Here's how the part is built. I have some questions about the finished solid (model axes, mm). A direction names the side the tool comes from. Round coordinates to 2 decimals unless told otherwise and drop trailing zeros. Order: outer loops, then holes, each group sorted by start corner. A loop starts at its lowest first (then second) coordinate and runs counter-clockwise, first axis right, second up. Notation, with made-up numbers: (17.5, 6.5) -> (46.5, 6.5) arc R13 cw to (46.5, 15.5) -> close; hole circle Ø7 at (70, 9). An arc over 180 degrees is marked (long way). Use a Markdown table: item, result. Add a question column.
(1) I want a section at D-D, the plane z = 25.5. Give the number of separate pieces and of enclosed holes in the cut face, then the cut area to 3 significant figures.
(2) On a 3-axis mill with a long thin cutter (end or side, diameter ignored), from which of +Z, -Z, +X, -X, +Y, -Y can I reach the whole of each face in a straight line? I mean faces 4 (the face through (7, 42, 28)), 5 (the face through (0, 32, 13)), 6 (the face through (2, 12, 28)), 7 (the face through (13, 36, 24)), 8 (the face through (5, 11, 14)). Say none if no direction works.
(3) I want a section at A-A, the plane z = 38. Please give me the cut outline in (x, y), then the cut area to 3 significant figures.
(4) Thinking about a two-plate mould opening in X: for faces 1 (the face through (2, 0, 14)), 2 (the face through (18.642, 25.535, 35.273)), 3 (the face through (15, 38, 26)), which applies, pulls with the +X half, pulls with the -X half, needs draft (parallel to the pull), parting line crosses it, or undercut?
(5) If I drill on probe 1 along Z at (x, y) = (3.95, 60); probe 2 along X at (y, z) = (26, 38); probe 3 along Z at (x, y) = (19, 25.45), over which ranges is the centre line in solid material (lowest first)?
(6) I want a section at B-B, the plane y = 60. Please give me the cut outline in (x, z).
(7) I want a section at C-C, the plane x = 20.5. Please give me the cut outline in (y, z), then the cut area to 3 significant figures.
(8) I'm going to push flat-ended pins straight in: P1, Ø11.5, axis at y = 14, z = 7, coming from the +X side; P2, Ø4, axis at x = 9, z = 24, coming from the -Y side; P3, Ø4, axis at x = 7.5, z = 19.5, coming from the +Y side. Where does each tip first touch, or does it pass through?
Autodesk Inventor part; units mm, degrees
ref_plane "YZ Plane" through (0, 0, 0) normal (1, 0, 0) x (0, 1, 0)
ref_plane "XZ Plane" through (0, 0, 0) normal (0, 1, 0) x (-1, 0, 0)
ref_plane "XY Plane" through (0, 0, 0) normal (0, 0, 1) x (1, 0, 0)
sketch "Sketch1" plane through (0, 0, 0) normal (1, 0, 0) x (0, 1, 0)
  line L0 (0, 0) -> (64, 0)
  line L1 (64, 0) -> (64, 28)
  line L2 (64, 28) -> (0, 28)
  line L3 (0, 28) -> (0, 0)
  line L4 (60, 24.5) -> (4, 24.5) construction
  line L5 (4, 24.5) -> (4, 3.5) construction
  line L6 (4, 3.5) -> (60, 3.5) construction
  line L7 (60, 3.5) -> (60, 24.5) construction
  line L8 (60, 24.5) -> (64, 24.5) construction
  line L9 (60, 24.5) -> (60, 28) construction
  line L10 (4, 3.5) -> (0, 3.5) construction
  line L11 (4, 3.5) -> (4, 0) construction
  circle A0 centre (60, 24.5) radius 2.6
  circle A1 centre (60, 3.5) radius 2.6
  circle A2 centre (4, 3.5) radius 2.6
  circle A3 centre (4, 24.5) radius 2.6
  dimension "d0" = 64
  dimension "d1" = 28
  dimension "d2" = 56
  dimension "d3" = 21
  dimension "d4" = 5.2
  dimension "d5" = 5.2
  dimension "d6" = 5.2
  dimension "d7" = 5.2
extrude "Extrusion1" add sketch "Sketch1" along normal blind 5
sketch "Sketch2" plane through (5, 0, 0) normal (1, 0, 0) x (0, 0, -1)
  line L0 (0, 0) -> (0, 64)
  line L1 (-28, 64) -> (-28, 0)
  line L2 (0, 23) -> (-28, 23)
  line L3 (-28, 23) -> (-28, 28)
  line L4 (-28, 28) -> (0, 28)
  line L5 (0, 28) -> (0, 23)
  line L6 (0, 64) -> (-28, 64)
  point P0 (0, 28)
  dimension "d10" = 41
  dimension "d11" = 5
extrude "Extrusion2" add sketch "Sketch2" along normal blind 20 contours L2 L1 L4 L0
sketch "Sketch3" plane through (0, 0, 28) normal (0, 0, 1) x (1, 0, 0)
  line L0 (5, 23) -> (25, 23)
  line L1 (0, 64) -> (0, 0)
  line L2 (25, 23) -> (0, 23)
  line L3 (0, 23) -> (0, 28)
  line L4 (0, 28) -> (25, 28)
  line L5 (25, 28) -> (25, 23)
  dimension "d14" = 5
extrude "Extrusion3" add sketch "Sketch3" along normal blind 20
sketch "Sketch4" plane through (0, 28, 48) normal (0, 1, 0) x (1, 0, 0)
  line L0 (0, 20) -> (0, 0) construction
  line L1 (0, 10) -> (25, 10) construction
  line L2 (25, 20) -> (25, 0) construction
  circle A0 centre (6, 10) radius 2.75
  circle A1 centre (19, 10) radius 2.75
  point P0 (0, 48)
  dimension "d20" = 5.5
  dimension "d21" = 5.5
  dimension "d22" = 6
  dimension "d24" = 6
extrude "Extrusion4" cut sketch "Sketch4" against normal up to next
sketch "Sketch7" plane through (5, 0, 0) normal (1, 0, 0) x (0, 0, -1)
  line L0 (-28, 28) -> (0, 28)
  line L1 (0, 28) -> (-4, 28)
  line L2 (-4, 28) -> (-4, 48)
  line L3 (-4, 48) -> (0, 48)
  line L4 (0, 48) -> (0, 28)
  line L5 (-28, 64) -> (-28, 28)
  line L6 (-28, 28) -> (-24, 28)
  line L7 (-24, 28) -> (-24, 48)
  line L8 (-24, 48) -> (-28, 48)
  line L9 (-28, 48) -> (-28, 28)
  point P0 (0, 0)
  dimension "d27" = 4
  dimension "d28" = 20
  dimension "d29" = 4
extrude "Extrusion5" add sketch "Sketch7" along normal blind 20
chamfer "Chamfer2" distance 20 angle 45 2 edges at (25, 48, 2) (25, 48, 26)
equation "\"d5\" = d4"
equation "\"d6\" = d4"
equation "\"d7\" = d4"
equation "\"d24\" = d22"
properties part number "X Axis Limit Switch Bracket"
Taken from the geometry:
| question | item | result |
|---|---|---|
| 1 | separate pieces | 3 |
| 1 | enclosed holes | 0 |
| 1 | area | 572 mm2 |
| 2 | face 4 | +Z, +X, -X, +Y |
| 2 | face 5 | +Z, -Z, -X, +Y, -Y |
| 2 | face 6 | +Z, +X, -X, -Y |
| 2 | face 7 | +X, +Y |
| 2 | face 8 | +Z, -Z, +X, -Y |
| 3 | outline | (0, 23) -> (3.25, 23) -> (3.25, 28) -> (0, 28) -> close; (8.75, 23) -> (16.25, 23) -> (16.25, 28) -> (8.75, 28) -> close; (21.75, 23) -> (25, 23) -> (25, 28) -> (21.75, 28) -> close |
| 3 | area | 70.0 mm2 |
| 4 | face 1 | needs draft |
| 4 | face 2 | undercut |
| 4 | face 3 | pulls with the +X half |
| 5 | probe 1 | z = 0 to 0.9, 6.1 to 21.9, 27.1 to 28 |
| 5 | probe 2 | x = 0 to 3.25, 8.75 to 16.25, 21.75 to 25 |
| 5 | probe 3 | z = 0 to 35.25, 40.75 to 48 |
| 6 | outline | (0, 0) -> (5, 0) -> (5, 0.9) -> (0, 0.9) -> close; (0, 6.1) -> (5, 6.1) -> (5, 21.9) -> (0, 21.9) -> close; (0, 27.1) -> (5, 27.1) -> (5, 28) -> (0, 28) -> close |
| 7 | outline | (23, 0) -> (32.5, 0) -> (32.5, 4) -> (28, 4) -> (28, 24) -> (32.5, 24) -> (32.5, 28) -> (28, 28) -> (28, 35.7) -> (23, 35.7) -> close; (23, 40.3) -> (28, 40.3) -> (28, 48) -> (23, 48) -> close |
| 7 | area | 253 mm2 |
| 8 | P1 | stops at x = 5 |
| 8 | P2 | stops at y = 23 |
| 8 | P3 | stops at y = 28 |
